Could you check a few things on this drawing? It's one solid part, dimensions in mm from its lowest x, y, z. A direction names the side the tool comes from. Give positions to 0.01 mm unless a question says otherwise; leave off trailing zeros. Order: outer loops, then holes, each group sorted by start corner. A loop starts at its lowest first (then second) coordinate and runs counter-clockwise, first axis right, second up. Notation, with made-up numbers: M -23.75,-3.75 L -5.75,-3.75 A16 cw -5.75,25.25 Z; hole C -33,88 d1. An arc over 180 degrees is marked long. One line per item, written item: value. Start each with the question number.
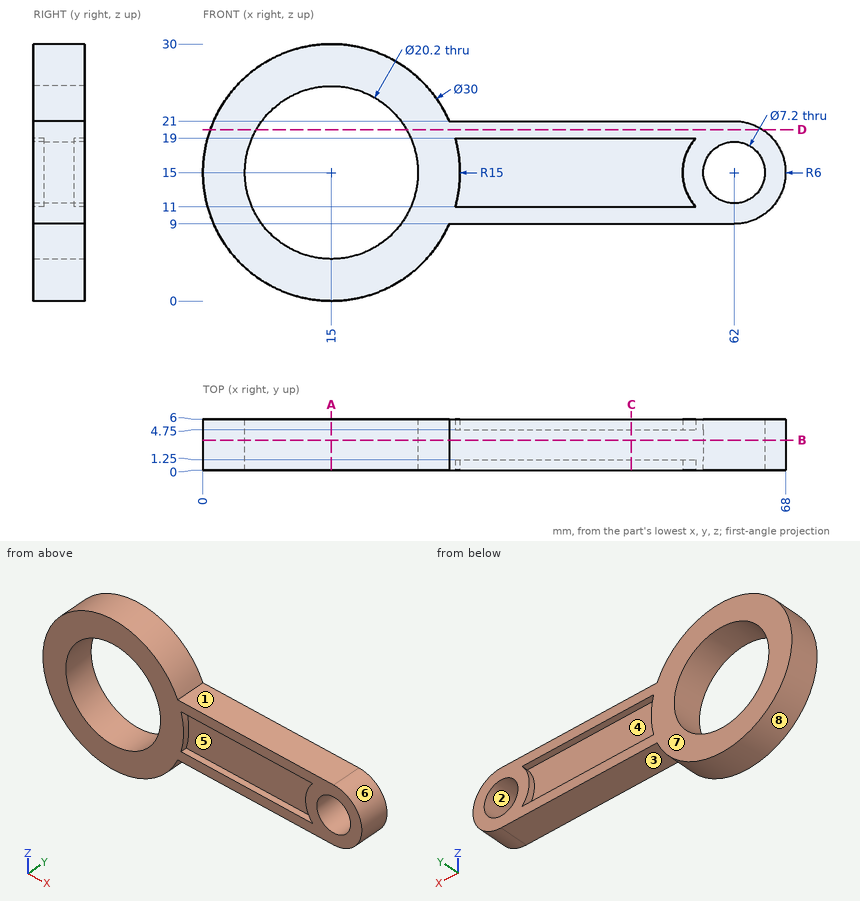
Item 1: Will these pins go through, and if not, where does the flat tip stop? P1, Ø3, axis at x = 46, y = 3, coming from the +Z side; P2, Ø1, axis at x = 38, y = 0.5, coming from the -Z side; P3, Ø2.5, axis at x = 42, z = 14.5, coming from the +Y side.
Item 2: I want a section at C-C on x = 50. Write out the boundary of the cut face in (y, z).
Item 3: Please list where these lines run through material, in increasing order: probe 1 along Z at (x, y) = (62, 2); probe 2 along Z at (x, y) = (51, 0.6); probe 3 along Y at (x, z) = (53, 16). Write a range as [from, to].
Item 4: I want a section at B-B on y = 3.55. Write out the boundary of the cut face in (x, z).
Item 5: For the marked faces 1, 2, 3 and 4, which set-ups out of +Z, -Z, +X, -X, +Y, -Y let a thin tool reach every point of the face, with its end or its side?
Item 6: I want a section at D-D on z = 20. Write out the boundary of the cut face in (x, y).
Item 7: I want a section at A-A on x = 15. Write out the boundary of the cut face in (y, z), plus the area to 3 significant figures.
Item 8: We'd pull the mould along X, two halves only. Please class the marked faces 5, 6, 7 and 8: +X half, -X half, draft (parallel to the pull), parting line (faces both ways), or undercut.
Answer below:
1. P1: stops at z = 21
1. P2: stops at z = 9
1. P3: stops at y = 4.75
2. outline: M 0,9 L 6,9 L 6,11 L 4.75,11 L 4.75,19 L 6,19 L 6,21 L 0,21 L 0,19 L 1.25,19 L 1.25,11 L 0,11 Z
3. probe 1: z = [9, 11.4], [18.6, 21]
3. probe 2: z = [9, 11], [19, 21]
3. probe 3: y = [1.25, 4.75]
4. outline: M 28.75,9 L 62,9 A6 ccw 62,21 L 28.75,21 A15 ccw long Z; hole C 15,15 d20.2; hole C 62,15 d7.2
5. face 1: +Z, +X, +Y, -Y
5. face 2: +Y, -Y
5. face 3: -Z, +X, +Y, -Y
5. face 4: +Y
6. outline: M 0.86,0 L 6.22,0 L 6.22,6 L 0.86,6 Z; M 23.78,0 L 65.32,0 L 65.32,6 L 23.78,6 Z
7. outline: M 0,0 L 6,0 L 6,4.9 L 0,4.9 Z; M 0,25.1 L 6,25.1 L 6,30 L 0,30 Z
7. area: 58.8 mm²
8. face 5: undercut
8. face 6: +X half
8. face 7: draft
8. face 8: parting line
